Here's the drawing with two shaded views (mm, measured from the low corner). I have some questions. A direction names the side the tool comes from. Coordinates: 2 decimals unless noted, no trailing zeros. Write each loop counter-clockwise with the first axis right and the second up, starting at its lowest first coordinate (ties: lowest second). Pieces come first, ordered by that corner, then holes. Notation, with made-up numbers: (43.25, 46.25) -> (95.25, 46.25) arc R26 ccw to (95.25, 66.25) -> close; hole circle Ø5 at (11, 8). An arc over 180 degrees is marked (long way). Use one line per item in the form item = value.
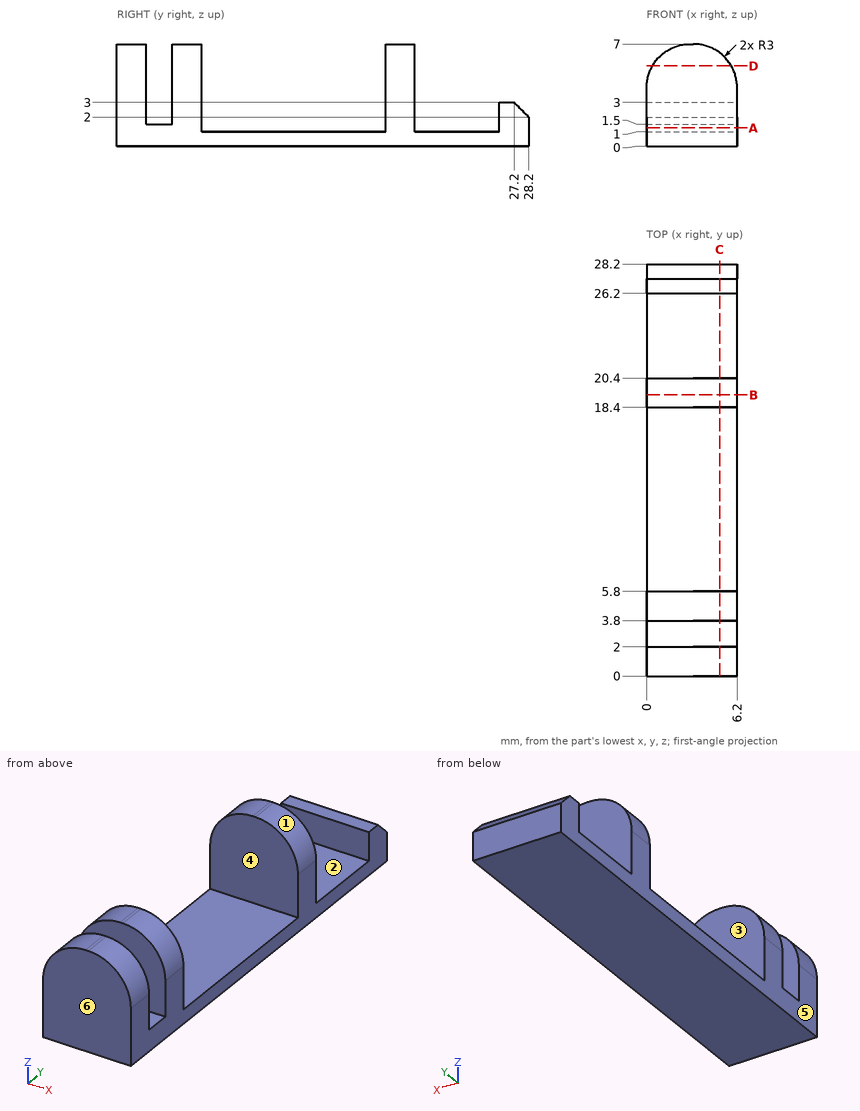
Q1. Suppose I cut it at D-D (z = 5.5). Write out the boundary of the cut face in (x, y), then the cut area to 3 significant figures.
Return value:
outline = (0.4, 0) -> (5.8, 0) -> (5.8, 2) -> (0.4, 2) -> close; (0.4, 3.8) -> (5.8, 3.8) -> (5.8, 5.8) -> (0.4, 5.8) -> close; (0.4, 18.4) -> (5.8, 18.4) -> (5.8, 20.4) -> (0.4, 20.4) -> close
area = 32.4 mm2
Q2. Suppose I cut it at A-A (z = 1.25). Write out the boundary of the cut face in (x, y), then the cut area to 3 significant figures.
Return value:
outline = (0, 0) -> (6.2, 0) -> (6.2, 5.8) -> (0, 5.8) -> close; (0, 18.4) -> (6.2, 18.4) -> (6.2, 20.4) -> (0, 20.4) -> close; (0, 26.2) -> (6.2, 26.2) -> (6.2, 28.2) -> (0, 28.2) -> close
area = 60.8 mm2
Q3. Suppose I cut it at C-C (x = 5). Write out the boundary of the cut face in (y, z).
Return value:
outline = (0, 0) -> (28.2, 0) -> (28.2, 2) -> (27.2, 3) -> (26.2, 3) -> (26.2, 1) -> (20.4, 1) -> (20.4, 6.4) -> (18.4, 6.4) -> (18.4, 1) -> (5.8, 1) -> (5.8, 6.4) -> (3.8, 6.4) -> (3.8, 1.5) -> (2, 1.5) -> (2, 6.4) -> (0, 6.4) -> close
Q4. Suppose I cut it at B-B (y = 19.25). Write out the boundary of the cut face in (x, z), then the cut area to 3 significant figures.
Return value:
outline = (0, 0) -> (6.2, 0) -> (6.2, 4) arc R3 ccw to (3.2, 7) -> (3, 7) arc R3 ccw to (0, 4) -> close
area = 39.5 mm2
Q5. For the marked faces 1 and 2, which set-ups out of +Z, -Z, +X, -X, +Y, -Y let a thin tool reach every point of the face, with its end or its side?
Return value:
face_1 = +Z, +X, +Y, -Y
face_2 = +Z, +X, -X
Q6. Will these pins go through, and if not, where does the flat tip stop? pin 1 (1.5 mm diameter, centred on x = 5.5, z = 4, fed in from +Y); pin 2 (0.5 mm diameter, centred on x = 4, y = 27, fed in from +Z); pin 3 (3 mm diameter, centred on x = 2, y = 11.5, fed in from +Z); pin 4 (3 mm diameter, centred on y = 17, z = 2, fed in from -X).
Return value:
pin_1 = 20.4
pin_2 = 3
pin_3 = 1
pin_4 = 0
Q7. Thinking about a two-plate mould opening in Y: for the marked faces 3, 4, 5 and 6, which applies, released by +Y, released by -Y, zero draft, split by the parting line, or undercut?
Return value:
face_3 = undercut
face_4 = undercut
face_5 = zero draft
face_6 = released by -Y
Q8. If I drill on line 1 (Y direction, x = 2, z = 6); line 2 (Y direction, x = 5, z = 2.5); line 3 (Y direction, x = 5.25, z = 2.25), over which ranges is the centre line in solid material (lowest first)? Write a range as from..to.
Return value:
line_1 = 0..2, 3.8..5.8, 18.4..20.4
line_2 = 0..2, 3.8..5.8, 18.4..20.4, 26.2..27.7
line_3 = 0..2, 3.8..5.8, 18.4..20.4, 26.2..27.95
